The listing builds one solid part. Answer for the finished solid, in the listing's coordinates (mm). Face numbers are marked on the shaded views. Coordinates: 2 decimals unless noted, no trailing zeros. Order: outer loops, then holes, each group sorted by start corner. A loop starts at its lowest first (then second) coordinate and runs counter-clockwise, first axis right, second up. Notation, with made-up numbers: M 14,-11.5 L 27,-11.5 A27 ccw 27,12.5 Z; hole C 30.5,29.5 d9. An arc over 180 degrees is marked long. One line per item, written item: value. Start each with the question number.
Q1. The part is cut by section A-A on x = 36.5. Give the vertices of the cut face in (y, z), then the cut area to 4 significant figures.
Q2. Determine the mould class of the marked faces 1, 2 and 3 for opening direction X: pulls with the +X half, pulls with the -X half, needs draft (parallel to the pull), parting line crosses it, or undercut.
Q3. Straight lines are drawn through the part: line 1 along Y through (x, z) = (26, 9.5); line 2 along Y through (x, z) = (11.5, 22.5). For each, find the intervals that lie inside material, in ascending order. Write a range as [from, to].
Q4. Each of these flat-tipped pins is pushed along its axis until it touches: pin 1 Ø8.5 at (x, z) = (7, 15) entering from +Y; pin 2 Ø6 at (x, y) = (-15.5, -5) entering from -Z; pin 3 Ø10.5 at (x, z) = (15.12, 15.97) entering from +Y. Where does it stop, or does it pass through?
```python
from build123d import *

# Parameters (mm, degrees)
SKETCH_W        = 95
SKETCH_H        = 24
PAD_DEPTH       = 33
SKETCH001_W     = 51
SKETCH001_H     = 29
POCKET_DEPTH    = 0.5
SKETCH002_R     = 7.5
POCKET001_DEPTH = 0.5
SKETCH003_R     = 4.5
HOLE_DEPTH      = 3
HOLE_TIPS_R     = 4.5


with BuildPart() as part:
    # Sketch → Pad (new body)
    with BuildSketch(Plane.XY):
        with Locations((14.785113, -6.63841)):
            Rectangle(SKETCH_W, SKETCH_H)
    extrude(amount=PAD_DEPTH)

    # Sketch001 (on Face4 of Pad) → Pocket (cut)
    with BuildSketch(Plane(origin=(0, 5.36159, 0), x_dir=(-1, 0, 0), z_dir=(0, 1, 0))):
        with Locations((-15.879372, 16.52663)):
            Rectangle(SKETCH001_W, SKETCH001_H)
    extrude(amount=-POCKET_DEPTH, mode=Mode.SUBTRACT)

    # Sketch002 (on Face11 of Pocket) → Pocket001 (cut)
    with BuildSketch(Plane(origin=(0, 4.86159, 0), x_dir=(-1, 0, 0), z_dir=(0, 1, 0))):
        with Locations((-15.141794, 16.087093)):
            Circle(SKETCH002_R)
    extrude(amount=-POCKET001_DEPTH, mode=Mode.SUBTRACT)

    # Sketch003 (on Face13 of Pocket001) → Hole (cut)
    with BuildSketch(Plane(origin=(0, 4.36159, 0), x_dir=(-1, 0, 0), z_dir=(0, 1, 0))):
        with Locations((-15.121763, 15.971645)):
            Circle(SKETCH003_R)
    extrude(amount=-HOLE_DEPTH, mode=Mode.SUBTRACT)

    # Hole tips → Hole tip 1 section 0
    with BuildSketch(Plane(origin=(0, 1.36159, 0), x_dir=(-1, 0, 0), z_dir=(0, 1, 0)), mode=Mode.PRIVATE) as hole_tip_1_s0:
        with Locations((-15.121763, 15.971645)):
            Circle(HOLE_TIPS_R)
    loft([hole_tip_1_s0.sketch, Vertex(15.121763, -1.342283, 15.971645)], mode=Mode.SUBTRACT)


solid = part.part
```
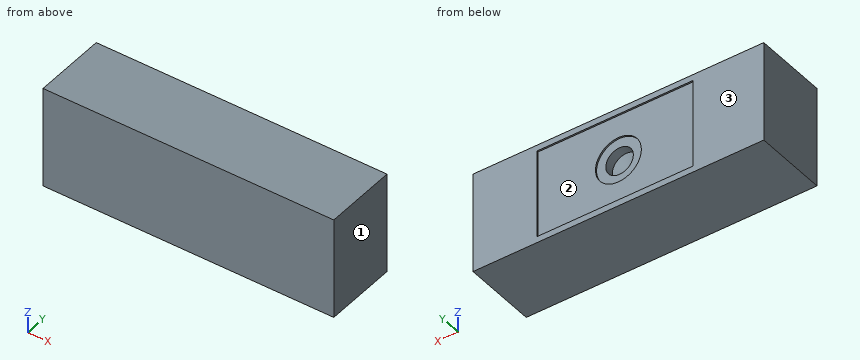
Output:
1. outline: M -18.64,0 L 5.36,0 L 5.36,2.03 L 4.86,2.03 L 4.86,31.03 L 5.36,31.03 L 5.36,33 L -18.64,33 Z
1. area: 777.5 mm^2
2. face 1: pulls with the +X half
2. face 2: undercut
2. face 3: needs draft
3. line 1: y = [-18.64, 4.86]
3. line 2: y = [-18.64, 4.36]
4. pin 1: stops at y = 4.86
4. pin 2: stops at z = 0
4. pin 3: stops at y = 4.36
